Model file for the job. Use its own axes, mm. Face numbers are marked on the shaded views. A direction names the side the tool comes from. Give positions to 0.01 mm unless a question says otherwise; leave off trailing zeros. Order: outer loops, then holes, each group sorted by start corner. A loop starts at its lowest first (then second) coordinate and runs counter-clockwise, first axis right, second up. Notation, with made-up numbers: (4.5, 46.25) -> (57.5, 46.25) arc R15 cw to (57.5, 52.25) -> close; hole circle Ø11 at (28, -3). An arc over 180 degrees is marked (long way). Answer in a Markdown table with one row per item. Add a question column.
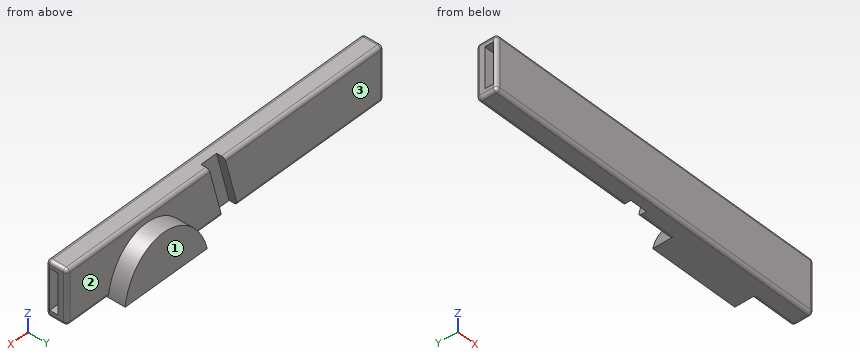
from build123d import *

# Parameters (mm, degrees)
SKETCH1_W               = 279.4
SKETCH1_H               = 63.5
BOSS_EXTRUDE1_DEPTH     = 12.7
BOSS_EXTRUDE2_DEPTH     = 50.8
SKETCH4_W               = 12.586648523787707
SKETCH4_H               = 6.172140988773259
CUT_EXTRUDE1_DEPTH      = 187.15064931818
CUT_EXTRUDE2_DEPTH      = 191.3909441326203
CUT_EXTRUDE2_DEPTH_BACK = 191.3909441326203
SKETCH5_W               = 77.64929915814443
SKETCH5_H               = 50.80000000000001
BOSS_EXTRUDE3_DEPTH     = 12.7
CUT_EXTRUDE4_DEPTH      = 57.15
CUT_EXTRUDE5_DEPTH      = 149.14020610558435
SKETCH23_W              = 260.35
SKETCH23_H              = 63.5
BOSS_EXTRUDE4_DEPTH     = 2.54
CUT_EXTRUDE6_DEPTH      = 149.37954115889764
SKETCH27_W              = 286.4591757611205
SKETCH27_H              = 45.03610752945451
CUT_EXTRUDE7_DEPTH      = 145.07085099474523
SKETCH31_W              = 40.63999999999999
SKETCH31_H              = 15.239999999999998
BOSS_EXTRUDE6_DEPTH     = 3.8099999999999996
CUT_EXTRUDE10_DEPTH     = 38.1
FILLET3_R               = 2.54


with BuildPart() as part:
    # Sketch1 → Boss-Extrude1 (new body)
    with BuildSketch(Plane(origin=(0, 0, 0), x_dir=(1, 0, 0), z_dir=(0, 1, 0))):
        Rectangle(SKETCH1_W, SKETCH1_H)
    extrude(amount=BOSS_EXTRUDE1_DEPTH)

    # Sketch2 → Boss-Extrude2 (add)
    with BuildSketch(Plane(origin=(0, 12.7, 0), x_dir=(1, 0, 0), z_dir=(0, 1, 0))):
        Polygon((-47.69999999999997, -21.749999999999986), (-28.33508326896288, -16.749999999999986), (-44.21008326896288, 44.733610621042764), (-63.57499999999998, 39.73361062104277), align=None)
        Polygon((8.514130017407421, 43.733610621042764), (24.389130017407417, -17.74999999999999), (43.7540467484445, -12.749999999999984), (27.879046748444473, 48.733610621042764), align=None)
    extrude(amount=BOSS_EXTRUDE2_DEPTH)

    # Sketch4 → Cut-Extrude1 (cut, through all)
    with BuildSketch(Plane(origin=(-13.591413263749278, 0, -52.63931722192361), x_dir=(-0.9682458365518543, 0, 0.24999999999999972), z_dir=(-0.24999999999999972, 0, -0.9682458365518543))):
        with Locations((6.706675646106144, 9.613929505613372)):
            Rectangle(SKETCH4_W, SKETCH4_H)
    extrude(amount=-CUT_EXTRUDE1_DEPTH, mode=Mode.SUBTRACT)

    # Sketch5 → Cut-Extrude2 (cut, two sides: drawn at the far end of the back side and taken through both)
    with BuildSketch(Plane(origin=(-30.618670005213612, 0, 7.905706600880859), x_dir=(-0.2500000000000001, 0, -0.9682458365518543), z_dir=(0.9682458365518541, 0, -0.25000000000000006)).offset(-CUT_EXTRUDE2_DEPTH_BACK)):
        with Locations((15.541003475924965, 38.1)):
            Rectangle(SKETCH5_W, SKETCH5_H)
    extrude(amount=CUT_EXTRUDE2_DEPTH + CUT_EXTRUDE2_DEPTH_BACK, mode=Mode.SUBTRACT)

    # Sketch6 → Boss-Extrude3 (add)
    with BuildSketch(Plane(origin=(0, 12.7, 0), x_dir=(1, 0, 0), z_dir=(0, 1, 0))):
        with BuildLine():
            Line((16.77527777661138, 35.78638852333846), (85.61472706482589, 47.625000000000014))
            add(Edge.make_bspline(
                [(16.77527777661138, 35.78638852333846), (24.308939625396, -8.020533750979865), (58.728664269503255, -2.101228012649095), (93.14838891361052, 3.8180777256816754), (85.61472706482589, 47.625000000000014)],
                knots=[4.71238898038469, 4.71238898038469, 4.71238898038469, 6.283185307179586, 6.283185307179586, 7.853981633974483, 7.853981633974483, 7.853981633974483], degree=2, weights=[1, 0.7071067811865476, 1, 0.7071067811865476, 1]))
        make_face()
    extrude(amount=BOSS_EXTRUDE3_DEPTH)

    # Sketch17 → Cut-Extrude4 (cut)
    with BuildSketch(Plane(origin=(139.70000000000002, 0, 0), x_dir=(0, 0, -1), z_dir=(1, 0, 0))):
        Polygon((26.670000000000012, -1.52e-15), (-3.80999999999998, -5.2e-15), (-3.80999999999998, 6.349999999999993), (26.670000000000012, 6.349999999999996), align=None)
    extrude(amount=-CUT_EXTRUDE4_DEPTH, mode=Mode.SUBTRACT)

    # Sketch22 → Cut-Extrude5 (cut, through all)
    with BuildSketch(Plane(origin=(0, 12.7, 0), x_dir=(1, 0, 0), z_dir=(0, 1, 0))):
        Polygon((139.70000000000002, -32.204899371851745), (120.65000000000002, -32.204899371851745), (120.65000000000002, 31.750000000000014), (139.70000000000005, 31.750000000000014), align=None)
    extrude(amount=-CUT_EXTRUDE5_DEPTH, mode=Mode.SUBTRACT)

    # Sketch23 → Boss-Extrude4 (add)
    with BuildSketch(Plane.XZ):
        with Locations((-9.524999999999963, -1.421e-14)):
            Rectangle(SKETCH23_W, SKETCH23_H)
    extrude(amount=BOSS_EXTRUDE4_DEPTH)

    # Sketch25 → Cut-Extrude6 (cut, through all)
    with BuildSketch(Plane.XZ.offset(-12.7)):
        with BuildLine():
            Line((86.05470968261828, -31.750000000000014), (17.622098670079023, -31.750000000000014))
            add(Edge.make_bspline(
                [(17.622098670079023, -31.750000000000014), (17.12530185096651, -33.75105992388856), (16.77527777661137, -35.78638852333846)],
                knots=[1.4779404098519116, 1.4779404098519116, 1.4779404098519116, 1.5707963267948968, 1.5707963267948968, 1.5707963267948968], degree=2, weights=[1, 0.9989224159229568, 1]))
            Line((16.77527777661137, -35.78638852333846), (85.6147270648259, -47.62500000000003))
            add(Edge.make_bspline(
                [(85.6147270648259, -47.62500000000003), (86.99136168467464, -39.620111142189245), (86.05470968261828, -31.750000000000014)],
                knots=[4.71238898038469, 4.71238898038469, 4.71238898038469, 5.073863183068598, 5.073863183068598, 5.073863183068598], degree=2, weights=[1, 0.9837114625910768, 1]))
        make_face()
    extrude(amount=-CUT_EXTRUDE6_DEPTH, mode=Mode.SUBTRACT)

    # Sketch27 → Cut-Extrude7 (cut, through all)
    with BuildSketch(Plane(origin=(0, 12.7, 0), x_dir=(1, 0, 0), z_dir=(0, 1, 0))):
        with Locations((-9.278901051751589, -31.408053764727235)):
            Rectangle(SKETCH27_W, SKETCH27_H)
    extrude(amount=-CUT_EXTRUDE7_DEPTH, mode=Mode.SUBTRACT)

    # Sketch31 → Boss-Extrude6 (add)
    with BuildSketch(Plane.ZY.offset(139.69999999999996)):
        with Locations((-11.430000000000017, 5.079999999999998)):
            Rectangle(SKETCH31_W, SKETCH31_H)
    extrude(amount=BOSS_EXTRUDE6_DEPTH)

    # Sketch32 → Cut-Extrude10 (cut)
    with BuildSketch(Plane.ZY.offset(143.50999999999996)):
        Polygon((-26.67000000000002, 6.35), (3.80999999999998, 6.35), (3.809999999999981, 0), (-26.67000000000002, 0), align=None)
    extrude(amount=-CUT_EXTRUDE10_DEPTH, mode=Mode.SUBTRACT)

    # Fillet3
    fillet3_edges = [part.edges().sort_by_distance(p)[0] for p in [
        (61.259240327968, 12.7, 8.889999999999981),
        (-77.32047702099145, 12.7, 8.889999999999983),
        (120.65000000000002, -2.54, -11.430000000000021),
        (-143.50999999999996, 5.079999999999999, 8.889999999999981),
        (-143.50999999999996, 5.08, -31.750000000000014),
        (120.65000000000002, 5.079999999999999, -31.750000000000014),
        (120.65000000000002, 5.08, 8.88999999999998),
        (-11.429999999999964, -2.54, -31.750000000000014),
        (-11.429999999999964, -2.54, 8.88999999999998),
        (-143.50999999999996, -2.54, -11.430000000000017),
        (120.65000000000002, 12.7, -11.430000000000014),
        (103.35235484130929, 12.7, -31.750000000000014),
        (4.49868822334534, 12.7, -31.750000000000014),
        (-143.50999999999996, 12.7, -11.430000000000016),
        (-82.56707846065376, 12.7, -31.750000000000014),
    ]]
    fillet(fillet3_edges, radius=FILLET3_R - 0.0001)  # a hair under: the kernel refuses the full size


solid = part.part
Item 1: Saw through at B-B on x = -32. List the corners of the cut face in (y, z).
Item 2: Wall check: line 1 (Y direction, x = 85.5, z = -9.5); line 2 (Y direction, x = 73.5, z = -1); line 3 (X direction, y = 2.5, z = -16.5). Give the ranges that are in metal, low to high.
Item 3: Which spindle directions (+Z, -Z, +X, -X, +Y, -Y) get a long thin tool onto all of the face, cutting with end or side? Do the marked faces 1, 2 and 3. Say none if no direction does.
Item 4: Pin check, flat tips, straight feed: pin 1 Ø10 at (x, y) = (-30, 12) entering from +Z; pin 2 Ø9 at (x, z) = (101.5, -12) entering from +Y; pin 3 Ø1.9 at (y, z) = (2, -15.5) entering from -X; pin 4 Ø2 at (y, z) = (20, -7) entering from +X. Stop position of each tip, or through.
Item 5: Saw through at A-A on x = -117. List the corners of the cut face in (y, z).
Evaluation:
| question | item | result |
|---|---|---|
| 1 | outline | (-2.54, -29.21) arc R2.54 ccw to (0, -31.75) -> (10.16, -31.75) arc R2.54 ccw to (12.7, -29.21) -> (12.7, 6.35) arc R2.54 ccw to (10.16, 8.89) -> (0, 8.89) arc R2.54 ccw to (-2.54, 6.35) -> close |
| 2 | line 1 | y = -2.54 to 0, 6.35 to 12.7 |
| 2 | line 2 | y = -2.54 to 12.7 |
| 2 | line 3 | x = -105.41 to 82.55 |
| 3 | face 1 | +Z, -Z, +X, -X, +Y |
| 3 | face 2 | +Z, +Y |
| 3 | face 3 | +Z, -Z, -X, +Y |
| 4 | pin 1 | stops at z = 8.89 |
| 4 | pin 2 | stops at y = 12.7 |
| 4 | pin 3 | stops at x = -105.41 |
| 4 | pin 4 | stops at x = 76.1 |
| 5 | outline | (-2.54, -29.21) arc R2.54 ccw to (0, -31.75) -> (10.16, -31.75) arc R2.54 ccw to (12.7, -29.21) -> (12.7, 6.35) arc R2.54 ccw to (10.16, 8.89) -> (0, 8.89) arc R2.54 ccw to (-2.54, 6.35) -> close; hole (0, -26.67) -> (6.35, -26.67) -> (6.35, 3.81) -> (0, 3.81) -> close |
